The model under review builds one solid part; all positions refer to its coordinate system, in mm. Give positions to 0.01 mm unless a question says otherwise; leave off trailing zeros. Order: outer loops, then holes, each group sorted by start corner. A loop starts at its lowest first (then second) coordinate and runs counter-clockwise, first axis right, second up.
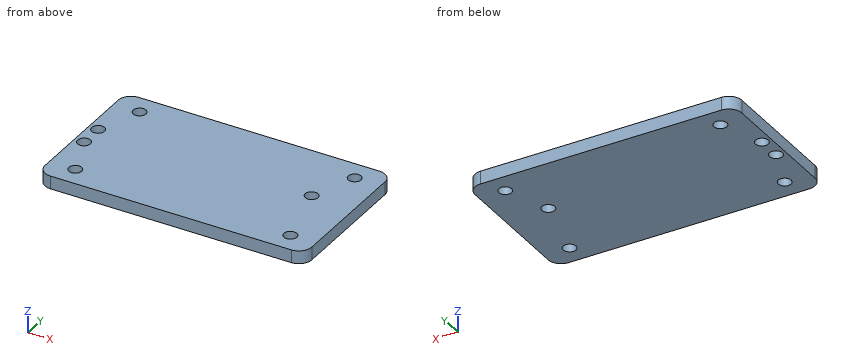
```python
from build123d import *

# Parameters (mm, degrees)
SKETCH1_R           = 1.5
BOSS_EXTRUDE1_DEPTH = 3


with BuildPart() as part:
    # Sketch1 → Boss-Extrude1 (new body)
    with BuildSketch(Plane.XY):
        with BuildLine():
            Line((-28, 17.5), (28, 17.5))
            ThreePointArc((28, 17.5), (30.121320344, 16.621320344), (31, 14.5))
            Line((31, 14.5), (31, -14.5))
            ThreePointArc((31, -14.5), (30.121320344, -16.621320344), (28, -17.5))
            Line((28, -17.5), (-28, -17.5))
            ThreePointArc((-28, -17.5), (-30.121320344, -16.621320344), (-31, -14.5))
            Line((-31, -14.5), (-31, 14.5))
            ThreePointArc((-31, 14.5), (-30.121320344, 16.621320344), (-28, 17.5))
        make_face()
        with Locations((-28.8, 2.8)):
            Circle(SKETCH1_R, mode=Mode.SUBTRACT)
        with Locations((-28.8, -2.8)):
            Circle(SKETCH1_R, mode=Mode.SUBTRACT)
        with Locations((21, 2.5)):
            Circle(SKETCH1_R, mode=Mode.SUBTRACT)
        with Locations((-25, 12.75)):
            Circle(SKETCH1_R, mode=Mode.SUBTRACT)
        with Locations((25, 12.75)):
            Circle(SKETCH1_R, mode=Mode.SUBTRACT)
        with Locations((25, -12.75)):
            Circle(SKETCH1_R, mode=Mode.SUBTRACT)
        with Locations((-25, -12.75)):
            Circle(SKETCH1_R, mode=Mode.SUBTRACT)
    extrude(amount=BOSS_EXTRUDE1_DEPTH)


solid = part.part
```
1. Take a section at B-B (z = 0.95). Write out the cut boundary in (x, y).
2. Take a section at D-D (y = -2). Write out the cut boundary in (x, z).
3. Take a section at A-A (y = -12.75). Write out the cut boundary in (x, z).
4. Take a section at C-C (x = 25). Write out the cut boundary in (y, z).
5. Insertion check: pin 1 (2.5 mm diameter, centred on x = -25, y = 12.75, fed in from -Z). The pin has a flat end and moves straight along its axis. Give the tip position at first contact, or say it passes through.
6. To check wall thickness, follow line 1 (Y direction, x = -25, z = 0.75); line 2 (Y direction, x = -28.8, z = 1.7); line 3 (X direction, y = -13, z = 2.75). State the ranges of each line that lie inside material, in increasing order.
Answer:
1. outline: (-31, -14.5) arc R3 ccw to (-28, -17.5) - (28, -17.5) arc R3 ccw to (31, -14.5) - (31, 14.5) arc R3 ccw to (28, 17.5) - (-28, 17.5) arc R3 ccw to (-31, 14.5) - close; hole circle Ø3 at (-28.8, -2.8); hole circle Ø3 at (-28.8, 2.8); hole circle Ø3 at (-25, -12.75); hole circle Ø3 at (-25, 12.75); hole circle Ø3 at (21, 2.5); hole circle Ø3 at (25, -12.75); hole circle Ø3 at (25, 12.75)
2. outline: (-31, 0) - (-30.07, 0) - (-30.07, 3) - (-31, 3) - close; (-27.53, 0) - (31, 0) - (31, 3) - (-27.53, 3) - close
3. outline: (-31, 0) - (-26.5, 0) - (-26.5, 3) - (-31, 3) - close; (-23.5, 0) - (23.5, 0) - (23.5, 3) - (-23.5, 3) - close; (26.5, 0) - (31, 0) - (31, 3) - (26.5, 3) - close
4. outline: (-17.5, 0) - (-14.25, 0) - (-14.25, 3) - (-17.5, 3) - close; (-11.25, 0) - (11.25, 0) - (11.25, 3) - (-11.25, 3) - close; (14.25, 0) - (17.5, 0) - (17.5, 3) - (14.25, 3) - close
5. pin 1: passes through
6. line 1: y = -17.5 to -14.25, -11.25 to 11.25, 14.25 to 17.5
6. line 2: y = -17.39 to -4.3, -1.3 to 1.3, 4.3 to 17.39
6. line 3: x = -31 to -26.48, -23.52 to 23.52, 26.48 to 31
